Input: part model. Units: mm. Frame: model coordinates. A direction names the side the tool comes from. Coordinates: 2 decimals unless noted, no trailing zeros. Loops run counter-clockwise (first coordinate to the right, second up) from the corner with the lowest first, then second, coordinate; pieces in that order, holes last. Notation, with made-up numbers: (68, 12.25) -> (101, 12.25) arc R15 ccw to (101, 21.25) -> close; hole circle Ø1 at (-7.5, 11). An arc over 180 degrees is marked (long way). Answer as a JSON object with one key per item and string values.
from build123d import *

# Parameters (mm, degrees)
SKETCH1_R           = 16.5
BOSS_EXTRUDE1_DEPTH = 6.5
BOSS_EXTRUDE1_TAPER = 8
SKETCH2_R           = 14.25
CUT_EXTRUDE1_DEPTH  = 4.5
CUT_EXTRUDE1_TAPER  = 21
CUT_EXTRUDE2_DEPTH  = 6
CHAMFER1_SIZE       = 1.5
SKETCH4_R           = 17.295094409
SKETCH4_R_2         = 14
CUT_EXTRUDE3_DEPTH  = 2


with BuildPart() as part:
    # Sketch1 → Boss-Extrude1 (new body)
    with BuildSketch(Plane(origin=(0, 0, 0), x_dir=(1, 0, 0), z_dir=(0, 1, 0))):
        Circle(SKETCH1_R)
    extrude(amount=BOSS_EXTRUDE1_DEPTH, taper=BOSS_EXTRUDE1_TAPER)

    # Sketch2 → Cut-Extrude1 (cut)
    with BuildSketch(Plane.XZ):
        Circle(SKETCH2_R)
    extrude(amount=-CUT_EXTRUDE1_DEPTH, taper=CUT_EXTRUDE1_TAPER, mode=Mode.SUBTRACT)

    # Sketch3 → Cut-Extrude2 (cut)
    with BuildSketch(Plane(origin=(0, 6.5, 0), x_dir=(1, 0, 0), z_dir=(0, 1, 0))):
        with BuildLine():
            Line((0, -12.5), (0, 12.5))
            ThreePointArc((0, 12.5), (12.5, 0), (0, -12.5))
        make_face()
    extrude(amount=-CUT_EXTRUDE2_DEPTH, mode=Mode.SUBTRACT)

    # Chamfer1
    chamfer1_edges = [part.edges().sort_by_distance(p)[0] for p in [
        (0, 4.5, 0),
    ]]
    chamfer(chamfer1_edges, length=CHAMFER1_SIZE)

    # Sketch4 → Cut-Extrude3 (cut)
    with BuildSketch(Plane(origin=(0, 6.5, 0), x_dir=(1, 0, 0), z_dir=(0, 1, 0))):
        Circle(SKETCH4_R)
        Circle(SKETCH4_R_2, mode=Mode.SUBTRACT)
    extrude(amount=-CUT_EXTRUDE3_DEPTH, mode=Mode.SUBTRACT)


solid = part.part
1. Line query: line 1 along Z through (x, y) = (0, 5.05); line 2 along X through (y, z) = (6, 0); line 3 along Y through (x, z) = (13.5, -6.5). Output: solid intervals per line, ascending.
Reply:
{"line 1": "z = -14 to -12.5, 12.5 to 14", "line 2": "x = -14 to 0, 12.5 to 14", "line 3": "y = 0 to 4.5"}
2. Access query for faces 1 (the face through (-3, 6.5, 0)), 2 (the face through (12.932, 5.514, 5.362)), 3 (the face through (-6, 4.5, 0)). Directions: +Z, -Z, +X, -X, +Y, -Y. A direction counts if a zero-diameter tool reaches every point of the face in a straight line with its end or side. Return the directions, or none.
Reply:
{"face 1": "+Z, -Z, +X, -X, +Y", "face 2": "+Y", "face 3": "-Y"}
3. Section query C-C (y = 3). Return loops of the section in (x, z), plus the area to 3 significant figures.
Reply:
{"outline": "circle Ø32.16 at (0, 0); hole circle Ø26.2 at (0, 0)", "area": "273 mm2"}
4. Mould query, pull axis Z, two halves, no side actions, for faces 4 (the face through (-14, 0, 5)), 5 (the face through (-1, 5, 0)), 6 (the face through (15.164, 4.282, -4.775)). Classes: pulls with the +Z half, pulls with the -Z half, needs draft (parallel to the pull), parting line crosses it, or undercut.
Reply:
{"face 4": "needs draft", "face 5": "undercut", "face 6": "parting line crosses it"}
5. Section query A-A (y = 0.5). Return loops of the section in (x, z), plus the area to 3 significant figures.
Reply:
{"outline": "circle Ø32.86 at (0, 0); hole circle Ø28.12 at (0, 0)", "area": "227 mm2"}
6. Pin query (flat end, axial travel): P1, Ø12.5, axis at x = 5, z = 2.5, coming from the -Y side; P2, Ø0.6, axis at y = 6.5, z = 0, coming from the +X side. Return the tip coordinate at first contact, or that it passes through.
Reply:
{"P1": "stops at y = 4.75", "P2": "stops at x = 14"}
7. Section query B-B (y = 5.25). Return loops of the section in (x, z).
Reply:
{"outline": "circle Ø28 at (0, 0); hole (-0.75, -12.48) arc R12.5 ccw (long way) to (-0.75, 12.48) -> close"}
